Geometry: final body of the model. Coordinates: model frame, mm. A direction names the side the tool comes from. Coordinates: 2 decimals unless noted, no trailing zeros. Write each loop counter-clockwise with the first axis right and the second up, starting at its lowest first coordinate (ties: lowest second). Pieces come first, ordered by that corner, then holes.
from build123d import *

# Parameters (mm, degrees)
SKETCH_1_R          = 2
EXTRUDE_1_DEPTH     = 2
SKETCH_4_W          = 8
SKETCH_4_H          = 2
EXTRUDE_3_DEPTH     = 15
SKETCH_5_R          = 1
CUT_EXTRUDE_1_DEPTH = 8
SKETCH_6_W          = 8
SKETCH_6_H          = 10
EXTRUDE_4_DEPTH     = 2
SKETCH_7_R          = 2
CUT_EXTRUDE_2_DEPTH = 2
FILLET_1_R          = 3
FILLET_2_R          = 2
SKETCH_9_R          = 3
CUT_EXTRUDE_3_DEPTH = 10


with BuildPart() as part:
    # 草图1 → 凸台-拉伸1 (new body)
    # profile 1 of 5: a face of its own
    with BuildSketch(Plane.XY):
        with BuildLine():
            Line((4, 6.34428877), (4, -6.34428877))
            ThreePointArc((4, -6.34428877), (6.566962768, -3.622844187), (7.5, 0))
            ThreePointArc((7.5, 0), (6.566962768, 3.622844187), (4, 6.34428877))
        make_face()
    # profile 2 of 5: a face of its own
    with BuildSketch(Plane.XY):
        with BuildLine():
            Line((-4, 6.34428877), (-4, -6.34428877))
            ThreePointArc((-4, -6.34428877), (0, -7.5), (4, -6.34428877))
            Line((4, -6.34428877), (4, 6.34428877))
            ThreePointArc((4, 6.34428877), (0, 7.5), (-4, 6.34428877))
        make_face()
        Circle(SKETCH_1_R, mode=Mode.SUBTRACT)
    # profile 3 of 5: a face of its own
    with BuildSketch(Plane.XY):
        with BuildLine():
            ThreePointArc((-4, 6.34428877), (-7.5, 0), (-4, -6.34428877))
            Line((-4, -6.34428877), (-4, 6.34428877))
        make_face()
    # profile 4 of 5: a face of its own
    with BuildSketch(Plane.XY):
        with BuildLine():
            Line((-4, 10), (-4, 6.34428877))
            ThreePointArc((-4, 6.34428877), (0, 7.5), (4, 6.34428877))
            Line((4, 6.34428877), (4, 10))
            Line((4, 10), (-4, 10))
        make_face()
    # profile 5 of 5: a face of its own
    with BuildSketch(Plane.XY):
        with BuildLine():
            Line((-4, -6.34428877), (-4, -10))
            Line((-4, -10), (4, -10))
            Line((4, -10), (4, -6.34428877))
            ThreePointArc((4, -6.34428877), (0, -7.5), (-4, -6.34428877))
        make_face()
    extrude(amount=EXTRUDE_1_DEPTH)

    # 草图4 → 凸台-拉伸3 (add)
    with BuildSketch(Plane.XY.offset(2)):
        with Locations((0, -11)):
            Rectangle(SKETCH_4_W, SKETCH_4_H)
        with Locations((0, 11)):
            Rectangle(SKETCH_4_W, SKETCH_4_H)
    extrude(amount=-EXTRUDE_3_DEPTH)

    # 草图5 → 切除-拉伸1 (cut)
    with BuildSketch(Plane(origin=(0, 0, 0), x_dir=(-1, 0, 0), z_dir=(0, 0, -1))):
        with Locations((0, 5.5)):
            Circle(SKETCH_5_R)
        with Locations((0, -5.5)):
            Circle(SKETCH_5_R)
    extrude(amount=-CUT_EXTRUDE_1_DEPTH, mode=Mode.SUBTRACT)

    # 草图6 → 凸台-拉伸4 (add)
    with BuildSketch(Plane(origin=(0, 0, -13), x_dir=(-1, 0, 0), z_dir=(0, 0, -1))):
        with Locations((0, -15)):
            Rectangle(SKETCH_6_W, SKETCH_6_H)
        with Locations((0, 15)):
            Rectangle(SKETCH_6_W, SKETCH_6_H)
    extrude(amount=EXTRUDE_4_DEPTH)

    # 草图7 → 切除-拉伸2 (cut)
    with BuildSketch(Plane.XY.offset(-13)):
        with Locations((0, 16)):
            Circle(SKETCH_7_R)
        with Locations((0, -16)):
            Circle(SKETCH_7_R)
    extrude(amount=-CUT_EXTRUDE_2_DEPTH, mode=Mode.SUBTRACT)

    # 圆角1
    fillet_1_edges = [part.edges().sort_by_distance(p)[0] for p in [
        (4, -6.34428877, 1),
        (-4, -6.34428877, 1),
        (-4, 6.34428877, 1),
        (4, 6.34428877, 1),
    ]]
    fillet(fillet_1_edges, radius=FILLET_1_R)

    # 圆角2
    fillet_2_edges = [part.edges().sort_by_distance(p)[0] for p in [
        (4, 20, -14),
        (-4, 20, -14),
        (4, -20, -14),
        (-4, -20, -14),
    ]]
    fillet(fillet_2_edges, radius=FILLET_2_R)

    # 草图9 → 切除-拉伸3 (cut)
    with BuildSketch(Plane.XY.offset(2)):
        Circle(SKETCH_9_R)
    extrude(amount=-CUT_EXTRUDE_3_DEPTH, mode=Mode.SUBTRACT)


solid = part.part
Item 1: Section C-C, the plane x = -0.25. State how many separate pieces and enclosed holes the cut face has, plus the area to 3 significant figures.
Derived:
separate pieces: 6
enclosed holes: 0
area: 104 mm2
Item 2: Set-up query: faces 1 (the flat face through (0, -12, -5)), 2 (the cylindrical face through (0.13, 6.49, 0.99)), 3 (the flat face through (-4, -11.8, -7.1)), 4 (the flat face through (4, -11.8, -7.1)), 5 (the flat face through (3.2, 0.1, 0)). Return all of +Z, -Z, +X, -X, +Y, -Y with unobstructed straight access to the full face (end or side cutting, diameter ignored); none if empty.
Derived:
face 1: +Z, +X, -X, -Y
face 2: +Z, -Z
face 3: +Z, -Z, -X, -Y
face 4: +Z, -Z, +X, -Y
face 5: -Z, +X, -X
Item 3: Section A-A, the plane y = -16. Output: boundary loops of the cut face in (x, z), plus the area to 3 significant figures.
Derived:
outline: (-4, -15) - (-2, -15) - (-2, -13) - (-4, -13) - close; (2, -15) - (4, -15) - (4, -13) - (2, -13) - close
area: 8.00 mm2
Item 4: Material intervals for probe 1 along Y at (x, z) = (0, 1.2); probe 2 along Y at (x, z) = (-1.75, -2.5); probe 3 along Z at (x, y) = (-3.5, 9.5), sorted ascending.
Derived:
probe 1: y = -12 to -6.5, -4.5 to -3, 3 to 4.5, 6.5 to 12
probe 2: y = -12 to -10, 10 to 12
probe 3: z = 0 to 2
Item 5: Pin query (flat end, axial travel): pin 1 (7.5 mm diameter, centred on x = -3.5, y = 4, fed in from -Z); pin 2 (1.8 mm diameter, centred on x = 0, y = -5.5, fed in from +Z); pin 3 (5 mm diameter, centred on y = -11, z = -4.5, fed in from -X); pin 4 (4 mm diameter, centred on x = 0.5, y = 18, fed in from +Z). Return the tip coordinate at first contact, or that it passes through.
Derived:
pin 1: stops at z = 0
pin 2: passes through
pin 3: stops at x = -4
pin 4: stops at z = -13
Item 6: Section B-B, the plane z = -3. Output: boundary loops of the cut face in (x, y), plus the area to 3 significant figures.
Derived:
outline: (-4, -12) - (4, -12) - (4, -10) - (-4, -10) - close; (-4, 10) - (4, 10) - (4, 12) - (-4, 12) - close
area: 32.0 mm2
Item 7: Pull-direction query (X, two-part tool) for faces 6 (the flat face through (2, 3, 2)), 7 (the cylindrical face through (-3, 0, 1)), 8 (the cylindrical face through (4.254, 6.618, 1.014)), 9 (the cylindrical face through (0, 18, -14)); classes: released by +X, released by -X, zero draft, split by the parting line, or undercut.
Derived:
face 6: zero draft
face 7: undercut
face 8: released by +X
face 9: undercut
Item 8: Section D-D, the plane x = 5.75. Output: boundary loops of the cut face in (y, z), plus the area to 3 significant figures.
Derived:
outline: (-4.82, 0) - (4.82, 0) - (4.82, 2) - (-4.82, 2) - close
area: 19.3 mm2
